Part model, mm, in its own coordinate system. A direction names the side the tool comes from. Coordinates: 2 decimals unless noted, no trailing zeros. Write each loop counter-clockwise with the first axis right and the second up, starting at its lowest first coordinate (ties: lowest second). Pieces come first, ordered by that corner, then holes. Notation, with made-up numbers: (50, 47) - (93, 47) arc R17 cw to (93, 62) - close; hole circle Ø1 at (10, 71). An arc over 180 degrees is marked (long way). Use a Markdown table: item, result.
```python
from build123d import *

# Parameters (mm, degrees)
F0_W     = 220
F0_H     = 6.6
F1_DEPTH = 1.9
F2_W     = 1.9
F2_H     = 6.6
F3_DEPTH = 20
F4_R     = 2


with BuildPart() as f1:
    # F0 (on Top) → F1 (new body)
    with BuildSketch(Plane.XY):
        with Locations((110, -3.3)):
            Rectangle(F0_W, F0_H)
    extrude(amount=F1_DEPTH)

    # F2 (on face) → F3 (join)
    with BuildSketch(Plane.XY.offset(1.9)):
        with Locations((219.05, -3.3)):
            Rectangle(F2_W, F2_H)
    extrude(amount=F3_DEPTH)

    # F4
    f4_edges = [f1.edges().sort_by_distance(p)[0] for p in [
        (220, -3.3, 0),
        (218.1, -3.3, 1.9),
        (219.05, -6.6, 21.9),
        (219.05, 0, 21.9),
        (0, -6.6, 0.95),
        (0, 0, 0.95),
    ]]
    fillet(f4_edges, radius=F4_R)


solid = f1.part
```
Item 1: Band-saw the part on B-B, the plane z = 11. Give the cut face in (x, y).
From the geometry:
| item | result |
|---|---|
| outline | (218.1, -6.6) - (220, -6.6) - (220, 0) - (218.1, 0) - close |
Item 2: Drop a flat-ended pin along its axis: P1, Ø2, axis at x = 152, y = -2.5, coming from the +Z side. Give the stop position or say it passes through.
From the geometry:
| item | result |
|---|---|
| P1 | z = 1.9 |
Item 3: Band-saw the part on C-C, the plane x = 185. Give the cut face in (y, z), then the cut area to 3 significant figures.
From the geometry:
| item | result |
|---|---|
| outline | (-6.6, 0) - (0, 0) - (0, 1.9) - (-6.6, 1.9) - close |
| area | 12.5 mm^2 |
Item 4: Which spindle directions (+Z, -Z, +X, -X, +Y, -Y) get a long thin tool onto all of the face, cutting with end or side? Do faces 1 (the face through (218.1, -3, 13)), 2 (the face through (110, -6.6, 1)). Say none if no direction does.
From the geometry:
| item | result |
|---|---|
| face 1 | +Z, -X, +Y, -Y |
| face 2 | +Z, -Z, +X, -X, -Y |
Item 5: Band-saw the part on A-A, the plane y = -3.5. Give the cut face in (x, z), then the cut area to 3 significant figures.
From the geometry:
| item | result |
|---|---|
| outline | (0, 0) - (218, 0) arc R2 ccw to (220, 2) - (220, 21.9) - (218.1, 21.9) - (218.1, 3.9) arc R2 cw to (216.1, 1.9) - (0, 1.9) - close |
| area | 456 mm^2 |
Item 6: Drill centre lines: probe 1 along X at (y, z) = (-0.25, 20.5); probe 2 along Z at (x, y) = (49.5, -5.5); probe 3 along X at (y, z) = (-4.25, 1). Where is each one in solid material? Low to high.
From the geometry:
| item | result |
|---|---|
| probe 1 | 218.1 to 220 |
| probe 2 | 0 to 1.9 |
| probe 3 | 0 to 219.73 |
